Autodesk Inventor part; units mm, degrees
ref_plane "YZ Plane" through (0, 0, 0) normal (1, 0, 0) x (0, 1, 0)
ref_plane "XZ Plane" through (0, 0, 0) normal (0, 1, 0) x (-1, 0, 0)
ref_plane "XY Plane" through (0, 0, 0) normal (0, 0, 1) x (1, 0, 0)
sketch "草圖1" plane through (0, 0, 0) normal (0, 1, 0) x (-1, 0, 0)
  line L0 (2.0138, -3.504) -> (-2.0277, -3.496)
  line L1 (-2.0277, -3.496) -> (-4.0414, 0.008)
  line L2 (-4.0414, 0.008) -> (-2.0138, 3.504)
  line L3 (-2.0138, 3.504) -> (2.0277, 3.496)
  line L4 (2.0277, 3.496) -> (4.0414, -0.008)
  line L5 (4.0414, -0.008) -> (2.0138, -3.504)
  point P0 (0, 0)
  point P1 (0, 0)
  dimension "d0" = 7
extrude "擠出1" add sketch "草圖1" along normal blind 3
sketch "草圖2" plane through (0, 3, 0) normal (0, 1, 0) x (1, 0, 0)
  circle A0 centre (0, 0) radius 2.5
  dimension "d3" = 5
extrude "擠出2" add sketch "草圖2" along normal blind 1.5
sketch "草圖3" plane through (0, 4.5, 0) normal (0, 1, 0) x (1, 0, 0)
  circle A0 centre (0, 0) radius 2.5
  circle A1 centre (0, 0) radius 3
  dimension "d7" = 6
extrude "擠出3" add sketch "草圖3" along normal blind 6 contours A0 | A1
sketch "草圖4" plane through (0, 0, 0) normal (0, -1, 0) x (1, 0, 0)
  circle A0 centre (0, 0) radius 1.9
  dimension "d11" = 3.8
extrude "擠出4" add sketch "草圖4" along normal blind 2 draft -35
sketch "草圖5" plane through (0, 10.5, 0) normal (0, 1, 0) x (1, 0, 0)
  circle A0 centre (0, 0) radius 3
hole "孔1" at (0, 10.5, 0) direction (0, -1, 0) diameter 2 depth 10.5 tip angle 118
chamfer "倒角1" distance 0.5 angle 45 3 edges at (-3, 4.5, 0) (-3, 10.5, 0) (0, 10.5, -1)
thread "螺紋1"
sketch "草圖6" plane through (0, -2, 0) normal (0, -1, 0) x (1, 0, 0)
  circle A0 centre (0, 0) radius 0.4996
hole "孔2" at (0, -2, 0) direction (0, 1, 0) diameter 0.4 end through all
sketch "草圖7" plane through (0, 10.5, 0) normal (0, 1, 0) x (1, 0, 0)
  circle A0 centre (0, 0) radius 1.5
hole "孔3" at (0, 10.5, 0) direction (0, -1, 0) diameter 1.5 depth 11.5 tip angle 118
properties part number "e3d_v6_nozzle"
Could you check a few things on this model? Use its own coordinates, in mm. A direction names the side the tool comes from. Give positions to 0.01 mm unless a question says otherwise; leave off trailing zeros. Order: outer loops, then holes, each group sorted by start corner. A loop starts at its lowest first (then second) coordinate and runs counter-clockwise, first axis right, second up. Notation, with made-up numbers: (-9.5, -2.75) -> (34.5, -2.75) arc R16 cw to (34.5, 27.25) -> close; hole circle Ø8 at (2.25, 62.25). An arc over 180 degrees is marked (long way). Answer in a Markdown table with one row per item. Add a question column.
Item 1: I'm going to push flat-ended pins straight in: P1, Ø2, axis at x = -0.5, z = 2, coming from the -Y side; P2, Ø2, axis at x = -3, z = -1, coming from the -Y side; P3, Ø2.5, axis at x = 0, z = 0, coming from the -Y side; P4, Ø2, axis at x = 2.5, z = -0.5, coming from the -Y side. Where does each tip first touch, or does it pass through?
Item 2: Please list where these lines run through material, in increasing order: probe 1 along X at (y, z) = (5.5, 0); probe 2 along Y at (x, z) = (3.25, 0.25).
Item 3: Imagine slicing it at C-C (y = 7). List the corners of the cut face in (x, z) for me, and give its area (3 significant figures).
Item 4: Imagine slicing it at B-B (y = 1). List the corners of the cut face in (x, z) for me.
Item 5: Imagine slicing it at D-D (y = 3.25). List the corners of the cut face in (x, z) for me, and give its area (3 significant figures).
Item 6: For faces 5 (the cylindrical face through (-0.03, -0.58, -0.75)), 6 (the flat face through (3.042, 1.479, 1.732)), which set-ups out of +Z, -Z, +X, -X, +Y, -Y let a thin tool reach every point of the face, with its end or its side?
Item 7: We'd pull the mould along Y, two halves only. Please class faces 1 (the cylindrical face through (-0.54, 3.74, -2.44)), 2 (the flat face through (-3, 3, 0)), 3 (the flat face through (-2, 0, 1)), 4 (the flat face through (-3.02, 1.48, 1.77)): pulls with the +Y half, pulls with the -Y half, needs draft (parallel to the pull), parting line crosses it, or undercut.
Result:
| question | item | result |
|---|---|---|
| 1 | P1 | y = -1.2 |
| 1 | P2 | y = 0 |
| 1 | P3 | y = -2 |
| 1 | P4 | y = -0.5 |
| 2 | probe 1 | -3 to -1, 1 to 3 |
| 2 | probe 2 | 0 to 3 |
| 3 | outline | circle Ø6 at (0, 0); hole circle Ø2 at (0, 0) |
| 3 | area | 25.1 mm2 |
| 4 | outline | (-4.04, -0.01) -> (-2.01, -3.5) -> (2.03, -3.5) -> (4.04, 0.01) -> (2.01, 3.5) -> (-2.03, 3.5) -> close; hole circle Ø2 at (0, 0) |
| 5 | outline | circle Ø5 at (0, 0); hole circle Ø2 at (0, 0) |
| 5 | area | 16.5 mm2 |
| 6 | face 5 | +Y |
| 6 | face 6 | +Z, +X, +Y, -Y |
| 7 | face 1 | undercut |
| 7 | face 2 | undercut |
| 7 | face 3 | pulls with the -Y half |
| 7 | face 4 | needs draft |
